from build123d import *

# Parameters (mm, degrees)
SKETCH1_R           = 55
BOSS_EXTRUDE1_DEPTH = 10
SKETCH2_R           = 4.25
CUT_EXTRUDE1_DEPTH  = 79.421935707
SKETCH3_R           = 0.75
CUT_EXTRUDE2_DEPTH  = 79.421935707
SKETCH4_R           = 32.75
SKETCH4_R_2         = 28.75
BOSS_EXTRUDE2_DEPTH = 3
CUT_EXTRUDE3_DEPTH  = 3
FILLET1_R           = 1.5
SKETCH6_R           = 1.75
CUT_EXTRUDE4_DEPTH  = 79.421935707
SKETCH7_R           = 5.125
CUT_EXTRUDE5_DEPTH  = 5
CIRPATTERN1_COUNT   = 4
CHAMFER1_SIZE       = 0.5


with BuildPart() as part:
    # Sketch1 → Boss-Extrude1 (new body)
    with BuildSketch(Plane(origin=(0, 0, 0), x_dir=(1, 0, 0), z_dir=(0, 1, 0))):
        with Locations(Location((0, 0, 0), (0, 0, 270))):
            Circle(SKETCH1_R)
    extrude(amount=BOSS_EXTRUDE1_DEPTH)

    # Sketch2 → Cut-Extrude1 (cut, through all)
    with BuildSketch(Plane(origin=(0, 10, 0), x_dir=(1, 0, 0), z_dir=(0, 1, 0))):
        with Locations(Location((0, 0, 0), (0, 0, 270))):
            Circle(SKETCH2_R)
    extrude(amount=-CUT_EXTRUDE1_DEPTH, mode=Mode.SUBTRACT)

    # Sketch3 → Cut-Extrude2 (cut, through all)
    with BuildSketch(Plane(origin=(0, 10, 0), x_dir=(1, 0, 0), z_dir=(0, 1, 0))):
        with Locations(Location((-20, 0, 0), (0, 0, 270))):
            Circle(SKETCH3_R)
        with Locations(Location((20, 0, 0), (0, 0, 270))):
            Circle(SKETCH3_R)
    extrude(amount=-CUT_EXTRUDE2_DEPTH, mode=Mode.SUBTRACT)

    # Sketch4 → Boss-Extrude2 (add)
    with BuildSketch(Plane(origin=(0, 10, 0), x_dir=(1, 0, 0), z_dir=(0, 1, 0))):
        with Locations(Location((0, 0, 0), (0, 0, 270))):
            Circle(SKETCH4_R)
        with Locations(Location((0, 0, 0), (0, 0, 270))):
            Circle(SKETCH4_R_2, mode=Mode.SUBTRACT)
    extrude(amount=BOSS_EXTRUDE2_DEPTH)

    # Sketch5 → Cut-Extrude3 (cut)
    with BuildSketch(Plane(origin=(0, 13, 0), x_dir=(1, 0, 0), z_dir=(0, 1, 0))):
        Polygon((-36.203629602, 26.304134665), (-26.304134665, 36.203629602), (0, 9.899494937), (26.527588401, 36.427083337), (36.427083337, 26.527588401), (9.899494937, 0), (37.563449253, -27.663954316), (27.663954316, -37.563449253), (0, -9.899494937), (-22.89121747, -32.790712406), (-32.790712406, -22.89121747), (-9.899494937, 0), align=None)
    extrude(amount=-CUT_EXTRUDE3_DEPTH, mode=Mode.SUBTRACT)

    # Fillet1
    fillet1_edges = [part.edges().sort_by_distance(p)[0] for p in [
        (-24.667284079, 11.5, 14.767789143),
        (-14.767789143, 11.5, 24.667284079),
        (14.767789143, 11.5, 24.667284079),
        (24.667284079, 11.5, 14.767789143),
        (24.667284079, 11.5, -14.767789143),
        (14.767789143, 11.5, -24.667284079),
        (-14.767789143, 11.5, -24.667284079),
        (-24.667284079, 11.5, -14.767789143),
        (-27.572330212, 11.5, -17.672835275),
        (-17.672835275, 11.5, -27.572330212),
        (17.672835275, 11.5, -27.572330212),
        (27.572330212, 11.5, -17.672835275),
        (27.572330212, 11.5, 17.672835275),
        (17.672835275, 11.5, 27.572330212),
        (-17.672835275, 11.5, 27.572330212),
        (-27.572330212, 11.5, 17.672835275),
    ]]
    fillet(fillet1_edges, radius=FILLET1_R)

    # Sketch6 → Cut-Extrude4 (cut, through all)
    with BuildSketch(Plane(origin=(0, 10, 0), x_dir=(1, 0, 0), z_dir=(0, 1, 0))):
        with Locations(Location((36.5, 0, 0), (0, 0, 270))):
            Circle(SKETCH6_R)
    cut_extrude4 = extrude(amount=-CUT_EXTRUDE4_DEPTH, mode=Mode.SUBTRACT)

    # Sketch7 → Cut-Extrude5 (cut)
    with BuildSketch(Plane.XZ):
        with Locations(Location((36.5, 0, 0), (0, 0, 270))):
            Circle(SKETCH7_R)
    cut_extrude5 = extrude(amount=-CUT_EXTRUDE5_DEPTH, mode=Mode.SUBTRACT)

    # CirPattern1: Cut-Extrude4, Cut-Extrude5 ×4 about axis
    cirpattern1_axis = Axis((0, 0, 0), (0, 1, 0))
    add([cut_extrude4.rotate(cirpattern1_axis, i * 360 / CIRPATTERN1_COUNT) for i in range(1, CIRPATTERN1_COUNT)], mode=Mode.SUBTRACT)
    add([cut_extrude5.rotate(cirpattern1_axis, i * 360 / CIRPATTERN1_COUNT) for i in range(1, CIRPATTERN1_COUNT)], mode=Mode.SUBTRACT)

    # Chamfer1
    chamfer1_edges = [part.edges().sort_by_distance(p)[0] for p in [
        (0, 0, -55),
    ]]
    chamfer(chamfer1_edges, length=CHAMFER1_SIZE)


solid = part.part
For this review, take the finished solid that the model builds, in its own axes (mm). A direction names the side the tool comes from. Coordinates: 2 decimals unless noted, no trailing zeros. Order: outer loops, then holes, each group sorted by start corner. A loop starts at its lowest first (then second) coordinate and runs counter-clockwise, first axis right, second up. Notation, with made-up numbers: (49, 15) -> (79, 15) arc R32 ccw to (79, 42) -> close; hole circle Ø5 at (-38, -35.75). An arc over 180 degrees is marked (long way). Return JSON: item names as keys, results as strings.
1. For line 1 (X direction, y = 8.25, z = 0); line 2 (X direction, y = 3.5, z = 0) (3 decimals); line 3 (Y direction, x = -32.5, z = 39), list the stretches that pass through material, from the lowest coordinate up. Write a range as from..to.
Answer block:
{"line 1": "-55..-38.25, -34.75..-20.75, -19.25..-4.25, 4.25..19.25, 20.75..34.75, 38.25..55", "line 2": "-55..-41.625, -31.375..-20.75, -19.25..-4.25, 4.25..19.25, 20.75..31.375, 41.625..55", "line 3": "0..10"}
2. The part is to be moulded in two halves that separate along Z. For faces 4 (the cylindrical face through (-27.461, 11.479, -16.742)), 5 (the cylindrical face through (0.38, 7.54, 34.79)), 6 (the flat face through (0, 13, -29)), say which applies: +Z half, -Z half, draft (parallel to the pull), parting line (faces both ways), or undercut.
Answer block:
{"face 4": "-Z half", "face 5": "undercut", "face 6": "draft"}
3. We need section B-B on x = 0. State how many separate pieces and enclosed holes the cut face has, and give its area (3 significant figures).
Answer block:
{"separate pieces": "4", "enclosed holes": "0", "area": "901 mm²"}
4. Machinability: for faces 1 (the cylindrical face through (-31.497, 2.465, -1.111)), 2 (the cylindrical face through (-32.75, 11.48, -0.23)), 3 (the flat face through (-11, 10, -1)), which of the approach directions +Z, -Z, +X, -X, +Y, -Y give a long, thin tool a straight path to every point of the face, cutting with its end or side? Answer none if there is none.
Answer block:
{"face 1": "-Y", "face 2": "-X, +Y", "face 3": "+Y"}
5. For pin 1 Ø4.5 at (x, z) = (36.5, 0) entering from +Y; pin 2 Ø3 at (x, z) = (38.5, 2) entering from -Y; pin 3 Ø1.5 at (x, y) = (29, 2) entering from -Z; pin 4 Ø3 at (x, z) = (0, -36.5) entering from +Y, all flat-tipped, find the tip position at first contact; note any pin that passes through.
Answer block:
{"pin 1": "y = 10", "pin 2": "y = 5", "pin 3": "z = -47.19", "pin 4": "through"}
6. We need section A-A on y = 1.75. Write out the cut boundary in (x, z) (3 decimals).
Answer block:
{"outline": "circle Ø110 at (0, 0); hole circle Ø10.25 at (-36.5, 0); hole circle Ø1.5 at (-20, 0); hole circle Ø10.25 at (0, -36.5); hole circle Ø10.25 at (0, 36.5); hole circle Ø8.5 at (0, 0); hole circle Ø1.5 at (20, 0); hole circle Ø10.25 at (36.5, 0)"}
